Part model, mm, in its own coordinate system. Round coordinates to 2 decimals unless told otherwise and drop trailing zeros. Loops run counter-clockwise (first coordinate to the right, second up) from the corner with the lowest first, then second, coordinate; pieces in that order, holes last.
1) Band-saw the part on A-A, the plane y = 54.25. Write the cut outline in (x, z), then the cut area to 3 significant figures.
2) Band-saw the part on B-B, the plane x = -107. Write the cut outline in (y, z) (3 decimals).
3) Band-saw the part on C-C, the plane z = 3. Write the cut outline in (x, y).
4) Drop a flat-ended pin along its axis: P1, Ø4, axis at x = -140.45, y = 52.93, coming from the +Z side (1 decimal). Give the stop position or say it passes through.
5) Probe line 1 (X direction, y = 51.25, z = 5.25); line 2 (X direction, y = 51, z = 3.25); line 3 (Y direction, x = -110.5, z = 2.5) (3 decimals). List the from-to ranges inside material, lowest first.
6) Band-saw the part on D-D, the plane y = 51. Write the cut outline in (x, z), then the cut area to 3 significant figures.
7) Mould opens along Y. For faces 1 (the flat face through (-125, 58.006, 3)), 2 (the cylindrical face through (-106.387, 51.965, 3.131)), 3 (the flat face through (-102.354, 53, 3)) say: +Y half, -Y half, draft (parallel to the pull), parting line (faces both ways), or undercut.
from build123d import *

# Parameters (mm, degrees)
SKETCH_1_W      = 44.45
SKETCH_1_H      = 9.525
SKETCH_1_R      = 2.50825
EXTRUDE_1_DEPTH = 6.35


with BuildPart() as part:
    # Эскиз1 → Бобышка-Вытянуть1 (new body)
    with BuildSketch(Plane.XY):
        with Locations((-124.578833131, 53.243233664)):
            Rectangle(SKETCH_1_W, SKETCH_1_H)
        with Locations((-108.703833131, 52.925733664)):
            Circle(SKETCH_1_R, mode=Mode.SUBTRACT)
        with Locations((-140.453833131, 52.925733664)):
            Circle(SKETCH_1_R, mode=Mode.SUBTRACT)
    extrude(amount=EXTRUDE_1_DEPTH)


solid = part.part
Reported:
1. outline: (-146.8, 0) - (-142.58, 0) - (-142.58, 6.35) - (-146.8, 6.35) - close; (-138.32, 0) - (-110.83, 0) - (-110.83, 6.35) - (-138.32, 6.35) - close; (-106.57, 0) - (-102.35, 0) - (-102.35, 6.35) - (-106.57, 6.35) - close
1. area: 228 mm2
2. outline: (48.481, 0) - (51.085, 0) - (51.085, 6.35) - (48.481, 6.35) - close; (54.766, 0) - (58.006, 0) - (58.006, 6.35) - (54.766, 6.35) - close
3. outline: (-146.8, 48.48) - (-102.35, 48.48) - (-102.35, 58.01) - (-146.8, 58.01) - close; hole circle Ø5.02 at (-140.45, 52.93); hole circle Ø5.02 at (-108.7, 52.93)
4. P1: passes through
5. line 1: x = -146.8 to -142.32, -138.59 to -110.57, -106.84 to -102.35
5. line 2: x = -146.8 to -142.06, -138.85 to -110.31, -107.1 to -102.35
5. line 3: y = 48.481 to 51.175, 54.676 to 58.006
6. outline: (-146.8, 0) - (-142.06, 0) - (-142.06, 6.35) - (-146.8, 6.35) - close; (-138.85, 0) - (-110.31, 0) - (-110.31, 6.35) - (-138.85, 6.35) - close; (-107.1, 0) - (-102.35, 0) - (-102.35, 6.35) - (-107.1, 6.35) - close
6. area: 241 mm2
7. face 1: +Y half
7. face 2: undercut
7. face 3: draft
